from build123d import *

# Parameters (mm, degrees)
SKETCH1_R           = 7.14375
BOSS_EXTRUDE1_DEPTH = 6.35
SKETCH2_R           = 10.16
BOSS_EXTRUDE2_DEPTH = 16.002
CHAMFER1_SIZE       = 0.254
SKETCH3_R           = 6.31825
BOSS_EXTRUDE3_DEPTH = 44.45
SKETCH5_R           = 6.35
BOSS_EXTRUDE4_DEPTH = 19.05
SKETCH11_R          = 6.31825
SKETCH11_R_2        = 5.5626
CUT_EXTRUDE2_DEPTH  = 16.51
CHAMFER2_SIZE       = 0.762
SKETCH8_W           = 1.016
SKETCH8_H           = 1.5875
SKETCH10_W          = 1.27
SKETCH10_H          = 3.175


with BuildPart() as part:
    # Sketch1 → Boss-Extrude1 (new body)
    with BuildSketch(Plane.XY):
        Circle(SKETCH1_R)
    extrude(amount=-BOSS_EXTRUDE1_DEPTH)

    # Sketch2 → Boss-Extrude2 (add)
    with BuildSketch(Plane.XY):
        Circle(SKETCH2_R)
    extrude(amount=BOSS_EXTRUDE2_DEPTH)

    # Chamfer1
    chamfer1_edges = [part.edges().sort_by_distance(p)[0] for p in [
        (-7.14375, 0, -6.35),
    ]]
    chamfer(chamfer1_edges, length=CHAMFER1_SIZE)

    # Sketch3 → Boss-Extrude3 (add)
    with BuildSketch(Plane.XY.offset(16.002)):
        Circle(SKETCH3_R)
    extrude(amount=BOSS_EXTRUDE3_DEPTH)

    # Sketch5 → Boss-Extrude4 (add)
    with BuildSketch(Plane(origin=(0, 0, -6.35), x_dir=(-1, 0, 0), z_dir=(0, 0, -1))):
        Circle(SKETCH5_R)
    extrude(amount=BOSS_EXTRUDE4_DEPTH)

    # Sketch11 → Cut-Extrude2 (cut)
    with BuildSketch(Plane.XY.offset(60.452)):
        Circle(SKETCH11_R)
        Circle(SKETCH11_R_2, mode=Mode.SUBTRACT)
    extrude(amount=-CUT_EXTRUDE2_DEPTH, mode=Mode.SUBTRACT)

    # Chamfer2
    chamfer2_edges = [part.edges().sort_by_distance(p)[0] for p in [
        (6.35, 0, -25.4),
        (-5.5626, 0, 60.452),
    ]]
    chamfer(chamfer2_edges, length=CHAMFER2_SIZE)

    # Sketch8 → Cut-Revolve3 (revolve, cut)
    with BuildSketch(Plane(origin=(0, 0, 0), x_dir=(1, 0, 0), z_dir=(0, 1, 0))):
        with Locations((-5.842, 7.14375)):
            Rectangle(SKETCH8_W, SKETCH8_H)
    revolve(axis=Axis((0, 0, 0), (0, 0, -1)), mode=Mode.SUBTRACT)

    # Sketch10 → Cut-Revolve4 (revolve, cut)
    with BuildSketch(Plane(origin=(0, 0, 0), x_dir=(1, 0, 0), z_dir=(0, 1, 0))):
        with Locations((-5.715, -42.3545)):
            Rectangle(SKETCH10_W, SKETCH10_H)
    revolve(axis=Axis((0, 0, 67.984878541), (0, 0, -1)), mode=Mode.SUBTRACT)


solid = part.part
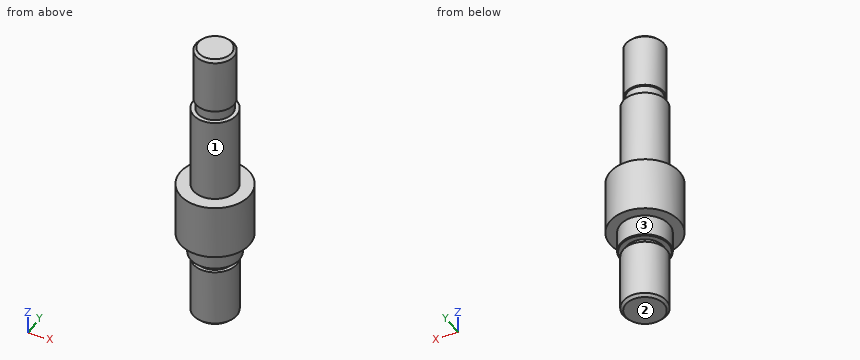
Could you check a few things on this model? Use its own coordinates, in mm. Face numbers are marked on the shaded views. A direction names the side the tool comes from. Round coordinates to 2 decimals unless told otherwise and drop trailing zeros. Order: outer loops, then holes, each group sorted by start corner. A loop starts at its lowest first (then second) coordinate and runs counter-clockwise, first axis right, second up.
(1) Imagine slicing it at D-D (z = 52). Write out the boundary of the cut face in (x, y).
Response values:
outline: circle Ø11.13 at (0, 0)
(2) Imagine slicing it at C-C (z = 28). Write out the boundary of the cut face in (x, y), plus the area to 3 significant figures.
Response values:
outline: circle Ø12.64 at (0, 0)
area: 125 mm2
(3) Please list where these lines run through material, in increasing order: line 1 along X through (y, z) = (-0.5, 14.5); line 2 along X through (y, z) = (8.5, 2); line 3 along Y through (x, z) = (0, 32).
Response values:
line 1: x = -10.15 to 10.15
line 2: x = -5.57 to 5.57
line 3: y = -6.32 to 6.32
(4) Which directions (+Z, -Z, +X, -X, +Y, -Y) give clear straight access to the entire face, cutting with the end or side of a thin tool? Please do the marked faces 1, 2 and 3.
Response values:
face 1: +Z
face 2: -Z, +X, -X, +Y, -Y
face 3: -Z
(5) I'm going to push flat-ended pins straight in: pin 1 (1.5 mm diameter, centred on x = 3, z = -7.5, fed in from +Y); pin 2 (10 mm diameter, centred on y = 2, z = 14.5, fed in from +X); pin 3 (1.5 mm diameter, centred on x = 7, y = -7.5, fed in from +Z); pin 4 (1.5 mm diameter, centred on y = -0.5, z = 42.5, fed in from -X). Where does each tip first touch, or does it pass through?
Response values:
pin 1: stops at y = 5.88
pin 2: stops at x = 10.16
pin 3: stops at z = 16
pin 4: stops at x = -5.08
